Build history of the part. All positions in model axes, mm. A direction names the side the tool comes from. Coordinates: 2 decimals unless noted, no trailing zeros. Order: outer loops, then holes, each group sorted by start corner. A loop starts at its lowest first (then second) coordinate and runs counter-clockwise, first axis right, second up. Notation, with made-up numbers: (67, 64.5) - (105, 64.5) arc R13 ccw to (105, 74.5) - close; hole circle Ø1 at (-23, 70.5). An arc over 180 degrees is marked (long way). Answer as CSV lines item,"result". Start each with the question number.
from build123d import *

# Parameters (mm, degrees)
ESQUISSE1_R             = 6
EXTRUSION1_DEPTH        = 5
ENL_V_MAT_EXTRU_1_DEPTH = 3
ESQUISSE3_W             = 3.158529234
ESQUISSE3_H             = 10.681133213
ENL_V_MAT_EXTRU_2_DEPTH = 10.848857802
ESQUISSE4_R             = 2
ENL_V_MAT_EXTRU_3_DEPTH = 9.366600265
CONG_1_R                = 0.1


with BuildPart() as part:
    # Esquisse1 → Extrusion1 (new body)
    with BuildSketch(Plane.XY):
        Circle(ESQUISSE1_R)
    extrude(amount=EXTRUSION1_DEPTH)

    # Esquisse2 → Enlèv. mat.-Extru.1 (cut)
    with BuildSketch(Plane.XY.offset(5)):
        Polygon((0, 4.041451884), (-3.5, 2.020725942), (-3.5, -2.020725942), (0, -4.041451884), (3.5, -2.020725942), (3.5, 2.020725942), align=None)
    extrude(amount=-ENL_V_MAT_EXTRU_1_DEPTH, mode=Mode.SUBTRACT)

    # Esquisse3 → Enlèv. mat.-Extru.2 (cut, through all)
    with BuildSketch(Plane.XY.offset(5)):
        with Locations((-6.579264617, 0.289330923)):
            Rectangle(ESQUISSE3_W, ESQUISSE3_H)
        with Locations((6.579264617, 0.289330923)):
            Rectangle(ESQUISSE3_W, ESQUISSE3_H)
    extrude(amount=-ENL_V_MAT_EXTRU_2_DEPTH, mode=Mode.SUBTRACT)

    # Esquisse4 → Enlèv. mat.-Extru.3 (cut, through all)
    with BuildSketch(Plane.XY.offset(2)):
        Circle(ESQUISSE4_R)
    extrude(amount=-ENL_V_MAT_EXTRU_3_DEPTH, mode=Mode.SUBTRACT)

    # Congé1
    cong_1_edges = [part.edges().sort_by_distance(p)[0] for p in [
        (0, 6, 0),
        (-5, 3.31662479, 2.5),
        (0, 6, 5),
        (5, 3.31662479, 2.5),
        (5, 0, 0),
        (0, -6, 0),
        (-5, 0, 0),
        (-2, 0, 0),
        (-5, 0, 5),
        (-5, -3.31662479, 2.5),
        (5, 0, 5),
        (0, -6, 5),
        (-1.75, 3.031088913, 5),
        (1.75, 3.031088913, 5),
        (-3.5, 0, 5),
        (3.5, 0, 5),
        (-1.75, -3.031088913, 5),
        (1.75, -3.031088913, 5),
        (5, -3.31662479, 2.5),
        (-2, 0, 2),
        (0, 4.041451884, 3.5),
        (-3.5, 2.020725942, 3.5),
        (-1.75, 3.031088913, 2),
        (3.5, 2.020725942, 3.5),
        (1.75, 3.031088913, 2),
        (-3.5, -2.020725942, 3.5),
        (-3.5, 0, 2),
        (3.5, -2.020725942, 3.5),
        (3.5, 0, 2),
        (0, -4.041451884, 3.5),
        (-1.75, -3.031088913, 2),
        (1.75, -3.031088913, 2),
    ]]
    fillet(cong_1_edges, radius=CONG_1_R)


solid = part.part
(1) Drop flat-ended pins along their axis: pin 1 Ø1.5 at (x, z) = (1.5, 1.5) entering from +Y; pin 2 Ø4.5 at (x, y) = (0, 0) entering from +Z. Give the stop position or say it passes through.
(2) Probe L1, parallel to Z at x = -1.5, y = -2; L2, parallel to X at y = 3.75, z = 4.05; L3, parallel to X at y = 1.5, z = 3.35. List the from-to ranges inside material, lowest first. Write a range as [from, to].
(3) Pull direction X, two halves, no side cores. Call faces 1 (the flat face through (-5, 0, 3)), 2 (the flat face through (-3.5, 0, 4)), 3 (the cylindrical face through (0, -6, 2)): +X half, -X half, draft (parallel to the pull), parting line (faces both ways), or undercut.
(4) Which spindle directions (+Z, -Z, +X, -X, +Y, -Y) get a long thin tool onto all of the face, cutting with end or side? Do faces 4 (the flat face through (3.5, 0, 4)), 5 (the flat face through (1, -4, 5)). Say none if no direction does.
(5) Band-saw the part on C-C on z = 2.65. List the corners of the cut face in (x, y), plus the area to 3 significant figures.
(6) Band-saw the part on A-A on y = 0. List the corners of the cut face in (x, z), plus the area to 3 significant figures.
(7) Band-saw the part on B-B on z = 0.55. List the corners of the cut face in (x, y), plus the area to 3 significant figures.
Filled in:
1,pin 1,"stops at y = 5.95"
1,pin 2,"stops at z = 2"
2,L1,"z = [0, 2]"
2,L2,"x = [-4.68, -0.5], [0.5, 4.68]"
2,L3,"x = [-5, -3.5], [3.5, 5]"
3,face 1,"-X half"
3,face 2,"undercut"
3,face 3,"parting line"
4,face 4,"+Z"
4,face 5,"+Z, +X, -X, +Y, -Y"
5,outline,"(-5, -3.29) arc R0.1 ccw to (-4.98, -3.34) arc R6 ccw to (4.98, -3.34) arc R0.1 ccw to (5, -3.29) - (5, 3.29) arc R0.1 ccw to (4.98, 3.34) arc R6 ccw to (-4.98, 3.34) arc R0.1 ccw to (-5, 3.29) - close; hole (-3.5, -1.96) arc R0.1 ccw to (-3.45, -2.05) - (-0.05, -4.01) arc R0.1 ccw to (0.05, -4.01) - (3.45, -2.05) arc R0.1 ccw to (3.5, -1.96) - (3.5, 1.96) arc R0.1 ccw to (3.45, 2.05) - (0.05, 4.01) arc R0.1 ccw to (-0.05, 4.01) - (-3.45, 2.05) arc R0.1 ccw to (-3.5, 1.96) - close"
5,area,"61.7 mm^2"
6,outline,"(-5, 0.1) arc R0.1 ccw to (-4.9, 0) - (-2.1, 0) arc R0.1 ccw to (-2, 0.1) - (-2, 1.9) arc R0.1 ccw to (-2.1, 2) - (-3.4, 2) arc R0.1 cw to (-3.5, 2.1) - (-3.5, 4.9) arc R0.1 ccw to (-3.6, 5) - (-4.9, 5) arc R0.1 ccw to (-5, 4.9) - close; (2, 0.1) arc R0.1 ccw to (2.1, 0) - (4.9, 0) arc R0.1 ccw to (5, 0.1) - (5, 4.9) arc R0.1 ccw to (4.9, 5) - (3.6, 5) arc R0.1 ccw to (3.5, 4.9) - (3.5, 2.1) arc R0.1 cw to (3.4, 2) - (2.1, 2) arc R0.1 ccw to (2, 1.9) - close"
6,area,"21.0 mm^2"
7,outline,"(-5, -3.29) arc R0.1 ccw to (-4.98, -3.34) arc R6 ccw to (4.98, -3.34) arc R0.1 ccw to (5, -3.29) - (5, 3.29) arc R0.1 ccw to (4.98, 3.34) arc R6 ccw to (-4.98, 3.34) arc R0.1 ccw to (-5, 3.29) - close; hole circle Ø4 at (0, 0)"
7,area,"91.5 mm^2"
